Here's how the part is built. I have some questions about the finished solid (model axes, mm). A direction names the side the tool comes from. Round coordinates to 2 decimals unless told otherwise and drop trailing zeros. Loops run counter-clockwise (first coordinate to the right, second up) from the corner with the lowest first, then second, coordinate; pieces in that order, holes last. Notation, with made-up numbers: M -12,64.25 L 14,64.25 A20 cw 14,94.25 Z; hole C 20,-2.5 d2. An arc over 180 degrees is marked long. Put each result on its own line as item: value. Start each with the question number.
```python
from build123d import *

# Parameters (mm, degrees)
F0_R     = 16.72
F1_DEPTH = 43
F2_R     = 16.72
F3_DEPTH = 43
F4_T     = 2


with BuildPart() as f1:
    # F0 (on Top) → F1 (new body, symmetric)
    with BuildSketch(Plane.XY):
        Circle(F0_R)
    extrude(amount=F1_DEPTH, both=True)

    # F2 (on Front) → F3 (join, symmetric)
    with BuildSketch(Plane.XZ):
        Circle(F2_R)
    extrude(amount=F3_DEPTH, both=True)

    # F4
    f4_openings = [f1.faces().sort_by_distance(p)[0] for p in [
        (0, 0, -43),
        (0, -43, 0),
        (0, 0, 43),
        (0, 43, 0),
    ]]
    offset(amount=F4_T, openings=f4_openings)


solid = f1.part
```
1) If I drill on probe 1 along Z at (x, y) = (0, -20); probe 2 along Y at (x, z) = (0, -17), over which ranges is the centre line in solid material (lowest first)? Write a range as from..to.
2) Suppose I cut it at C-C (z = -3). Write out the boundary of the cut face in (x, y), plus the area to 3 significant figures.
3) I'm going to push flat-ended pins straight in: P1, Ø5, axis at y = -10.5, z = 27, coming from the -X side; P2, Ø8, axis at x = -1, y = 14, coming from the -Z side; P3, Ø6, axis at y = 10.5, z = -32, coming from the -X side; P4, Ø1.5, axis at x = 11, y = 22.5, coming from the -Z side. Where does each tip first touch, or does it pass through?
4) Suppose I cut it at A-A (x = -2.5). Write out the boundary of the cut face in (y, z), plus the area to 3 significant figures.
5) Suppose I cut it at D-D (x = 15.5). Write out the boundary of the cut face in (y, z).
6) If we mould it in two halves opening along X, with no side actions, what happens to faces 4 (the face through (-7.021, 15.341, 43)), 5 (the face through (-13.27, -10.17, -25.98)), 6 (the face through (-13.8, 12.65, -25.98))? For each: pulls with the +X half, pulls with the -X half, needs draft (parallel to the pull), parting line crosses it, or undercut.
7) Suppose I cut it at B-B (y = -10). Write out the boundary of the cut face in (x, z).
8) On a 3-axis mill with a long thin cutter (end or side, diameter ignored), from which of +Z, -Z, +X, -X, +Y, -Y can I reach the whole of each face in a straight line? I mean faces 1 (the face through (8.638, -16.608, 26.579)), 2 (the face through (-13.8, 25.98, 12.65)), 3 (the face through (8.638, -26.579, -16.608)). Say none if no direction works.
Results are:
1. probe 1: -18.72..-16.72, 16.72..18.72
1. probe 2: -43..-16.72, 16.72..43
2. outline: M -18.48,-43 L -16.45,-43 L -16.45,-3 A16.72 cw -16.45,3 L -16.45,43 L -18.48,43 L -18.48,3 A18.72 ccw -18.48,-3 Z; M 16.45,-43 L 18.48,-43 L 18.48,-3 A18.72 ccw 18.48,3 L 18.48,43 L 16.45,43 L 16.45,3 A16.72 cw 16.45,-3 Z
2. area: 349 mm²
3. P1: x = -16.92
3. P2: z = -43
3. P3: x = -17.15
3. P4: z = -15.66
4. outline: M -43,-18.55 L -18.55,-18.55 L -18.55,-43 L -16.53,-43 L -16.53,-16.53 L -43,-16.53 Z; M -43,16.53 L -16.53,16.53 L -16.53,43 L -18.55,43 L -18.55,18.55 L -43,18.55 Z; M 16.53,-43 L 18.55,-43 L 18.55,-18.55 L 43,-18.55 L 43,-16.53 L 16.53,-16.53 Z; M 16.53,16.53 L 43,16.53 L 43,18.55 L 18.55,18.55 L 18.55,43 L 16.53,43 Z
4. area: 411 mm²
5. outline: M -43,-10.5 L -10.5,-10.5 L -10.5,-43 L -6.27,-43 L -6.27,-6.27 L -43,-6.27 Z; M -43,6.27 L -6.27,6.27 L -6.27,43 L -10.5,43 L -10.5,10.5 L -43,10.5 Z; M 6.27,-43 L 10.5,-43 L 10.5,-10.5 L 43,-10.5 L 43,-6.27 L 6.27,-6.27 Z; M 6.27,6.27 L 43,6.27 L 43,10.5 L 10.5,10.5 L 10.5,43 L 6.27,43 Z
6. face 4: needs draft
6. face 5: undercut
6. face 6: parting line crosses it
7. outline: M -15.83,-43 L -13.4,-43 L -13.4,-10 A16.72 cw -13.4,10 L -13.4,43 L -15.83,43 L -15.83,10 A18.72 ccw -15.83,-10 Z; M 13.4,-43 L 15.83,-43 L 15.83,-10 A18.72 ccw 15.83,10 L 15.83,43 L 13.4,43 L 13.4,10 A16.72 cw 13.4,-10 Z
8. face 1: +Z
8. face 2: +Y
8. face 3: -Y
